Verification items for the finished model (mm, model axes). Face numbers are marked on the shaded views. A direction names the side the tool comes from. Round coordinates to 2 decimals unless told otherwise and drop trailing zeros. Order: outer loops, then holes, each group sorted by start corner. A loop starts at its lowest first (then second) coordinate and runs counter-clockwise, first axis right, second up. Notation, with made-up numbers: (-18.5, -38) -> (38.5, -38) arc R27 cw to (38.5, -2) -> close; hole circle Ø3 at (57.25, 24). An arc over 180 degrees is marked (long way). Answer in a Markdown table with one row per item. Add a question column.
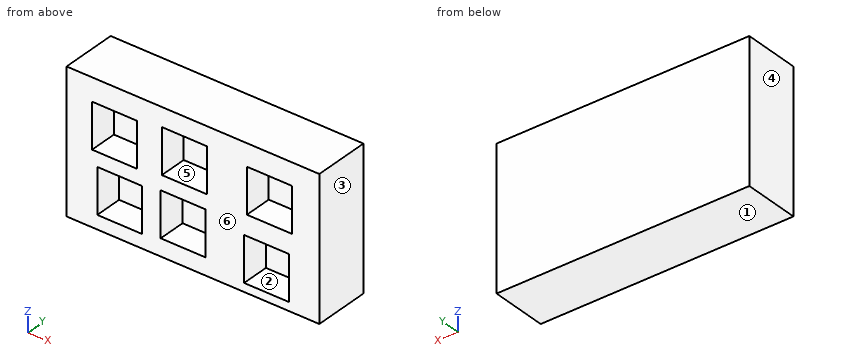
```python
from build123d import *

# Parameters (mm, degrees)
F0_W     = 114.3
F0_H     = 63.5
F1_DEPTH = 25.4
F2_W     = 20.32
F2_H     = 20.32
F3_DEPTH = 12.573


with BuildPart() as f1:
    # F0 (on Front) → F1 (new body)
    with BuildSketch(Plane.XZ):
        Rectangle(F0_W, F0_H)
    extrude(amount=F1_DEPTH)

    # F2 (on face) → F3 (cut, symmetric)
    with BuildSketch(Plane.XZ.offset(25.4)):
        with Locations((-35.47241, 11.268726)):
            Rectangle(F2_W, F2_H)
        with Locations((-3.90384, 13.083012)):
            Rectangle(F2_W, F2_H)
        with Locations((34.559014, 11.631584)):
            Rectangle(F2_W, F2_H)
        with Locations((-33.113839, -15.401271)):
            Rectangle(F2_W, F2_H)
        with Locations((33.289013, -17.759843)):
            Rectangle(F2_W, F2_H)
        with Locations((-4.423103, -13.882415)):
            Rectangle(F2_W, F2_H)
    extrude(amount=F3_DEPTH, both=True, mode=Mode.SUBTRACT)


solid = f1.part
```
1) Thickness scan on L1, parallel to X at y = -16.5, z = 4.5; L2, parallel to Z at x = -27.5, y = -16.25; L3, parallel to Z at x = -3, y = -23. Record the ranges inside material, lowest first. Write a range as [from, to].
2) Draft check along X on the marked faces 3, 4, 5 and 6. Enter one of: +X half, -X half, draft (parallel to the pull), parting line (faces both ways), or undercut.
3) Cross-section at A-A, the plane x = -11.5. Record the boundary of the cut face in (y, z).
4) Tool access check on the marked faces 1 and 2. Record the directions out of +Z, -Z, +X, -X, +Y, -Y that give a thin tool (end or side, any length) a straight path to the whole face; none if there is none.
5) Depth check by flat-ended pin: P1, Ø6, axis at x = 29.5, z = -16, coming from the -Y side. Enter the tip coordinate at first touch or a pass-through.
6) Cross-section at C-C, the plane z = -15. Record the boundary of the cut face in (x, y).
7) Cross-section at B-B, the plane y = -18. Record the boundary of the cut face in (x, z).
Results below:
| question | item | result |
|---|---|---|
| 1 | L1 | [-57.15, -45.63], [-25.31, -14.06], [6.26, 24.4], [44.72, 57.15] |
| 1 | L2 | [-31.75, -25.56], [-5.24, 1.11], [21.43, 31.75] |
| 1 | L3 | [-31.75, -24.04], [-3.72, 2.92], [23.24, 31.75] |
| 2 | face 3 | +X half |
| 2 | face 4 | -X half |
| 2 | face 5 | undercut |
| 2 | face 6 | draft |
| 3 | outline | (-25.4, -31.75) -> (0, -31.75) -> (0, 31.75) -> (-25.4, 31.75) -> (-25.4, 23.24) -> (-12.83, 23.24) -> (-12.83, 2.92) -> (-25.4, 2.92) -> (-25.4, -3.72) -> (-12.83, -3.72) -> (-12.83, -24.04) -> (-25.4, -24.04) -> close |
| 4 | face 1 | -Z, +X, -X, +Y, -Y |
| 4 | face 2 | -Y |
| 5 | P1 | y = -12.83 |
| 6 | outline | (-57.15, -25.4) -> (-43.27, -25.4) -> (-43.27, -12.83) -> (-22.95, -12.83) -> (-22.95, -25.4) -> (-14.58, -25.4) -> (-14.58, -12.83) -> (5.74, -12.83) -> (5.74, -25.4) -> (23.13, -25.4) -> (23.13, -12.83) -> (43.45, -12.83) -> (43.45, -25.4) -> (57.15, -25.4) -> (57.15, 0) -> (-57.15, 0) -> close |
| 7 | outline | (-57.15, -31.75) -> (57.15, -31.75) -> (57.15, 31.75) -> (-57.15, 31.75) -> close; hole (-45.63, 1.11) -> (-25.31, 1.11) -> (-25.31, 21.43) -> (-45.63, 21.43) -> close; hole (-43.27, -25.56) -> (-22.95, -25.56) -> (-22.95, -5.24) -> (-43.27, -5.24) -> close; hole (-14.58, -24.04) -> (5.74, -24.04) -> (5.74, -3.72) -> (-14.58, -3.72) -> close; hole (-14.06, 2.92) -> (6.26, 2.92) -> (6.26, 23.24) -> (-14.06, 23.24) -> close; hole (23.13, -27.92) -> (43.45, -27.92) -> (43.45, -7.6) -> (23.13, -7.6) -> close; hole (24.4, 1.47) -> (44.72, 1.47) -> (44.72, 21.79) -> (24.4, 21.79) -> close |
